```python
from build123d import *

# Parameters (mm, degrees)
F0_W      = 19.05
F0_H      = 19.05
F1_DEPTH  = 12.7
F2_R      = 3.96875
F3_DEPTH  = 12.701
F12_DEPTH = 19.05


with BuildPart() as f1:
    # F0 (on Top) → F1 (new body)
    with BuildSketch(Plane.XY):
        with Locations((-9.525, 9.525)):
            Rectangle(F0_W, F0_H)
    extrude(amount=F1_DEPTH)

    # F2 (on face) → F3 (cut, through all)
    with BuildSketch(Plane.XY.offset(12.7)):
        with Locations((-9.525, 9.525)):
            Circle(F2_R)
    extrude(amount=-F3_DEPTH, mode=Mode.SUBTRACT)

    # F7: sweep along a path in F4
    with BuildLine(Plane.XY.offset(12.7)) as f7_path:
        CenterArc((-9.525, 9.525), 9.525, 0, 360)
    # F6 (on mid) → F7 (sweep, cut)
    with BuildSketch(Plane.XZ.offset(-9.525)):
        Polygon((-24.6209054321, 11.966576386), (-19.05, 12.7), (-24.6209054321, 13.433423614), align=None)
    sweep(path=f7_path.line, mode=Mode.SUBTRACT)

    # F9 (on mid) → F10 (revolve, cut)
    with BuildSketch(Plane.XZ.offset(-9.525)):
        Polygon((8.2884986839, 0), (0, 0), (8.2884986839, -1.091201553), align=None)
        Polygon((8.2884986839, 1.091201553), (0, 0), (8.2884986839, 0), align=None)
    revolve(axis=Axis((-9.525, 9.525, 12.7), (0, 0, 1)), mode=Mode.SUBTRACT)

    # F11 (on face) → F12 (cut)
    with BuildSketch(Plane.XZ):
        Polygon((0, 7.62), (-1.27, 6.35), (0, 5.08), align=None)
    extrude(amount=-F12_DEPTH, mode=Mode.SUBTRACT)


solid = f1.part
```
Part model, mm, in its own coordinate system. A direction names the side the tool comes from. Round coordinates to 2 decimals unless told otherwise and drop trailing zeros. Answer in a Markdown table with one row per item. Add a question column.
Q1. 3-axis set-ups, long thin cutter, end or side, ignore diameter. For faces 1 (the face through (-10, 19.05, 6)), 2 (the face through (-0.64, 9.39, 5.72)): which of +Z, -Z, +X, -X, +Y, -Y reach the whole face in a straight line?
Q2. Mould opens along X. For faces 3 (the face through (-7.7, 6, 6.4)), 4 (the face through (-2.152, 2.098, 12.576)), 5 (the face through (-19.05, 9, 6)), 6 (the face through (-10, 0, 6)) say: +X half, -X half, draft (parallel to the pull), parting line (faces both ways), or undercut.
Q3. Wall check: L1, parallel to Z at x = -0.75, y = 10.25; L2, parallel to X at y = 6, z = 6.75; L3, parallel to X at y = 7.75, z = 2. Give the ranges that are in metal, low to high. Write a range as from..to.
Q4. Pin check, flat tip, straight feed: pin 1 (10.5 mm diameter, centred on x = -9.525, y = 9.525, fed in from -Z). Stop position of the tip, or through.
Established:
| question | item | result |
|---|---|---|
| 1 | face 1 | +Z, -Z, +X, -X, +Y |
| 1 | face 2 | +X, +Y, -Y |
| 2 | face 3 | undercut |
| 2 | face 4 | +X half |
| 2 | face 5 | -X half |
| 2 | face 6 | draft |
| 3 | L1 | z = 0..5.83, 6.87..12.7 |
| 3 | L2 | x = -19.05..-11.35, -7.7..-0.87 |
| 3 | L3 | x = -19.05..-13.07, -5.98..0 |
| 4 | pin 1 | stops at z = 0 |
